Check sheet for the drawn part. Datum: minimum x, y, z corner. Units: mm. A direction names the side the tool comes from. Coordinates: 2 decimals unless noted, no trailing zeros. Write each loop counter-clockwise with the first axis right and the second up, starting at its lowest first coordinate (ties: lowest second). Pieces come first, ordered by that corner, then holes. Notation, with made-up numbers: (-8.5, -1.5) -> (20.5, -1.5) arc R14 cw to (20.5, 19.5) -> close; hole circle Ø9 at (-31.5, 35). An arc over 180 degrees is marked (long way). Answer in a Markdown table with one row per item.
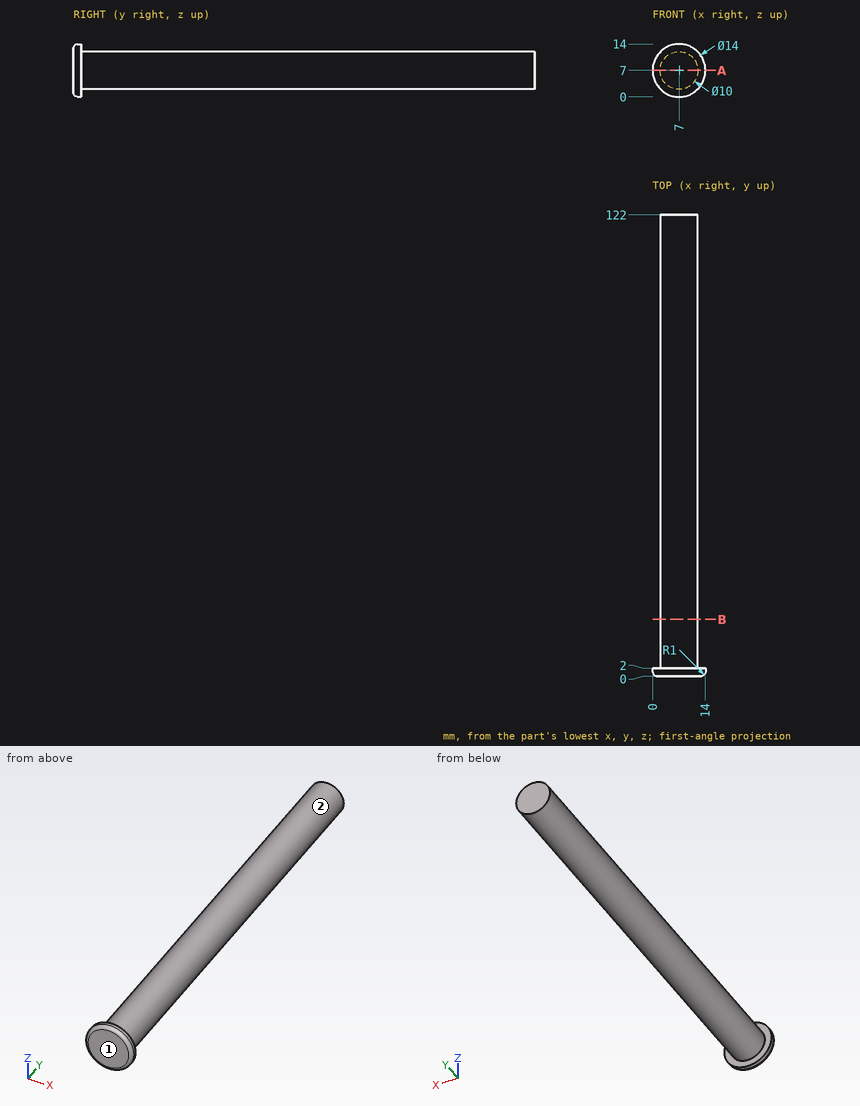
1. Access from +Z, -Z, +X, -X, +Y, -Y to the whole of each face (thin tool, end or side, straight path). Record for the marked faces 1 and 2.
Findings below:
| item | result |
|---|---|
| face 1 | +Z, -Z, +X, -X, -Y |
| face 2 | +Y |
2. Go/stop test with flat-tipped pins: pin 1 (4 mm diameter, centred on x = 8.5, y = 108.5, fed in from +Z); pin 2 (2 mm diameter, centred on y = 92, z = 10, fed in from +X); pin 3 (2 mm diameter, centred on y = 45.5, z = 7.5, fed in from -X). Record where each tip stops, or that it passes through.
Findings below:
| item | result |
|---|---|
| pin 1 | stops at z = 12 |
| pin 2 | stops at x = 11.58 |
| pin 3 | stops at x = 2 |
3. Sectioned sample at B-B, the plane y = 15. Record the cut outline in (x, z).
Findings below:
| item | result |
|---|---|
| outline | circle Ø10 at (7, 7) |
4. Sectioned sample at A-A, the plane z = 7. Record the cut outline in (x, y).
Findings below:
| item | result |
|---|---|
| outline | (0, 1) arc R1 ccw to (1, 0) -> (13, 0) arc R1 ccw to (14, 1) -> (14, 2) -> (12, 2) -> (12, 122) -> (2, 122) -> (2, 2) -> (0, 2) -> close |
5. Material ranges on probe 1 along X at (y, z) = (6, 6.75); probe 2 along Y at (x, z) = (13, 7.5), recorded low to high. Write a range as from..to.
Findings below:
| item | result |
|---|---|
| probe 1 | x = 2.01..11.99 |
| probe 2 | y = 0..2 |
